The model under review builds one solid part; all positions refer to its coordinate system, in mm. A direction names the side the tool comes from. Coordinates: 2 decimals unless noted, no trailing zeros. Order: outer loops, then holes, each group sorted by start corner. A loop starts at its lowest first (then second) coordinate and runs counter-clockwise, first axis right, second up. Notation, with made-up numbers: (-9, -39.5) -> (5, -39.5) arc R13 ccw to (5, -27.5) -> close; hole circle Ø5 at (87, -24.5). An arc over 180 degrees is marked (long way). Answer as CSV lines item,"result". Start each with the question number.
from build123d import *
from OCP.BRepFilletAPI import BRepFilletAPI_MakeChamfer

# Parameters (mm, degrees)
SKETCH1_W           = 60
SKETCH1_H           = 45
BOSS_EXTRUDE1_DEPTH = 30
SKETCH2_W           = 8
SKETCH2_H           = 16
CUT_EXTRUDE1_DEPTH  = 20
CHAMFER1_SIZE       = 15
CHAMFER1_SIZE2      = 1.312329953
CHAMFER2_SIZE       = 5
CHAMFER2_SIZE2      = 5.958767963
CUT_EXTRUDE2_DEPTH  = 10


with BuildPart() as part:
    # Sketch1 → Boss-Extrude1 (new body)
    with BuildSketch(Plane(origin=(0, 0, 0), x_dir=(1, 0, 0), z_dir=(0, 1, 0))):
        with Locations((-30, 22.5)):
            Rectangle(SKETCH1_W, SKETCH1_H)
    extrude(amount=BOSS_EXTRUDE1_DEPTH)

    # Sketch2 → Cut-Extrude1 (cut)
    with BuildSketch(Plane(origin=(0, 0, 0), x_dir=(-1, 0, 0), z_dir=(0, -1, 0))):
        with Locations((47, 21)):
            Rectangle(SKETCH2_W, SKETCH2_H)
        with Locations((13, 21)):
            Rectangle(SKETCH2_W, SKETCH2_H)
    extrude(amount=-CUT_EXTRUDE1_DEPTH, mode=Mode.SUBTRACT)

    # Chamfer1: one chamfer whose edges measure the first distance from different faces: ONE call of the kernel's chamfer builder (chamfer() names one face for all edges)
    chamfer1_edges_1 = [part.edges().sort_by_distance(p)[0] for p in [
        (-51, 20, -21),
    ]]
    chamfer1_side_1 = [part.faces().sort_by_distance(p)[0] for p in [
        (-51, 10, -21),
    ]]
    chamfer1_edges_2 = [part.edges().sort_by_distance(p)[0] for p in [
        (-43, 20, -21),
    ]]
    chamfer1_side_2 = [part.faces().sort_by_distance(p)[0] for p in [
        (-43, 10, -21),
    ]]
    chamfer1_edges_3 = [part.edges().sort_by_distance(p)[0] for p in [
        (-17, 20, -21),
    ]]
    chamfer1_side_3 = [part.faces().sort_by_distance(p)[0] for p in [
        (-17, 10, -21),
    ]]
    chamfer1_edges_4 = [part.edges().sort_by_distance(p)[0] for p in [
        (-9, 20, -21),
    ]]
    chamfer1_side_4 = [part.faces().sort_by_distance(p)[0] for p in [
        (-9, 10, -21),
    ]]
    chamfer1 = BRepFilletAPI_MakeChamfer(part.part.solid().wrapped)
    for e in chamfer1_edges_1:
        chamfer1.Add(CHAMFER1_SIZE, CHAMFER1_SIZE2, e.wrapped, chamfer1_side_1[0].wrapped)  # the first distance lies on this face
    for e in chamfer1_edges_2:
        chamfer1.Add(CHAMFER1_SIZE, CHAMFER1_SIZE2, e.wrapped, chamfer1_side_2[0].wrapped)  # the first distance lies on this face
    for e in chamfer1_edges_3:
        chamfer1.Add(CHAMFER1_SIZE, CHAMFER1_SIZE2, e.wrapped, chamfer1_side_3[0].wrapped)  # the first distance lies on this face
    for e in chamfer1_edges_4:
        chamfer1.Add(CHAMFER1_SIZE, CHAMFER1_SIZE2, e.wrapped, chamfer1_side_4[0].wrapped)  # the first distance lies on this face
    add(Compound.cast(chamfer1.Shape()), mode=Mode.REPLACE)

    # Chamfer2: one chamfer whose edges measure the first distance from different faces: ONE call of the kernel's chamfer builder (chamfer() names one face for all edges)
    chamfer2_edges_1 = [part.edges().sort_by_distance(p)[0] for p in [
        (-13, 20, -29),
    ]]
    chamfer2_side_1 = [part.faces().sort_by_distance(p)[0] for p in [
        (-13, 9.298544625, -29),
    ]]
    chamfer2_edges_2 = [part.edges().sort_by_distance(p)[0] for p in [
        (-13, 20, -13),
    ]]
    chamfer2_side_2 = [part.faces().sort_by_distance(p)[0] for p in [
        (-13, 9.298544625, -13),
    ]]
    chamfer2_edges_3 = [part.edges().sort_by_distance(p)[0] for p in [
        (-47, 20, -29),
    ]]
    chamfer2_side_3 = [part.faces().sort_by_distance(p)[0] for p in [
        (-47, 9.298544625, -29),
    ]]
    chamfer2_edges_4 = [part.edges().sort_by_distance(p)[0] for p in [
        (-47, 20, -13),
    ]]
    chamfer2_side_4 = [part.faces().sort_by_distance(p)[0] for p in [
        (-47, 9.298544625, -13),
    ]]
    chamfer2 = BRepFilletAPI_MakeChamfer(part.part.solid().wrapped)
    for e in chamfer2_edges_1:
        chamfer2.Add(CHAMFER2_SIZE, CHAMFER2_SIZE2, e.wrapped, chamfer2_side_1[0].wrapped)  # the first distance lies on this face
    for e in chamfer2_edges_2:
        chamfer2.Add(CHAMFER2_SIZE, CHAMFER2_SIZE2, e.wrapped, chamfer2_side_2[0].wrapped)  # the first distance lies on this face
    for e in chamfer2_edges_3:
        chamfer2.Add(CHAMFER2_SIZE, CHAMFER2_SIZE2, e.wrapped, chamfer2_side_3[0].wrapped)  # the first distance lies on this face
    for e in chamfer2_edges_4:
        chamfer2.Add(CHAMFER2_SIZE, CHAMFER2_SIZE2, e.wrapped, chamfer2_side_4[0].wrapped)  # the first distance lies on this face
    add(Compound.cast(chamfer2.Shape()), mode=Mode.REPLACE)

    # Sketch4 → Cut-Extrude2 (cut)
    with BuildSketch(Plane(origin=(0, 0, -45), x_dir=(-1, 0, 0), z_dir=(0, 0, -1))):
        with BuildLine():
            Line((10, 0), (28.5, 0))
            ThreePointArc((28.5, 0), (34.073421984, 6.184666101), (42.397874378, 6.313583642))
            ThreePointArc((42.397874378, 6.313583642), (46.400635454, 7.606885175), (45.740315255, 11.761244612))
            ThreePointArc((45.740315255, 11.761244612), (24.568698428, 15.91316533), (10, 0))
        make_face()
    extrude(amount=-CUT_EXTRUDE2_DEPTH, mode=Mode.SUBTRACT)


solid = part.part
1) Consider section A-A (y = 8.25). Give the boundary of the cut face in (x, z).
2) Mouldability with a two-part tool opening along Y and no side actions: class faces 4 (the face through (-33.965, 6.134, -40.07)), 5 (the face through (-12.956, 17.535, -25.979)), 6 (the face through (-28, 9, -35)), 7 (the face through (-60, 15, -22)) as released by +Y, released by -Y, zero draft, split by the parting line, or undercut.
3) Wall thickness on L1, parallel to X at y = 7.5, z = -27; L2, parallel to Y at x = -11, z = -20; L3, parallel to Z at x = -49, y = 2.5: over which ranges is each line inside the solid? List them lowest first. Write a range as [from, to].
4) Tool access review of faces 1 (the face through (-30, 15, 0)), 2 (the face through (-46.367, 7.553, -40.07)), 3 (the face through (-51, 2, -21)): name each direction out of +Z, -Z, +X, -X, +Y, -Y from which nothing blocks a thin tool from reaching the whole face with its end or side.
5) Insertion check: pin 1 Ø3 at (x, y) = (-35, 9.5) entering from -Z. The pin has a flat end and moves straight along its axis. Give the tip position at first contact, or say it passes through.
6) Consider section D-D (z = -15.5). Give the boundary of the cut face in (x, y).
7) Consider section C-C (x = -35). Give the boundary of the cut face in (y, z), plus the area to 3 significant figures.
8) Consider section B-B (z = -20). Give the boundary of the cut face in (x, y), plus the area to 3 significant figures.
Result:
1,outline,"(-60, -45) -> (-46.7, -45) -> (-46.7, -35) -> (-13.86, -35) -> (-13.86, -45) -> (0, -45) -> (0, 0) -> (-60, 0) -> close; hole (-50.72, -29) -> (-43.28, -29) -> (-43.28, -13) -> (-50.72, -13) -> close; hole (-16.72, -29) -> (-9.28, -29) -> (-9.28, -13) -> (-16.72, -13) -> close"
2,face 4,"undercut"
2,face 5,"released by -Y"
2,face 6,"undercut"
2,face 7,"zero draft"
3,L1,"[-60, -50.78], [-43.22, -16.78], [-9.22, 0]"
3,L2,"[20, 30]"
3,L3,"[-45, -29], [-13, 0]"
4,face 1,"+Z, +X, -X, +Y, -Y"
4,face 2,"-Z"
4,face 3,"-Y"
5,pin 1,"z = -35"
6,outline,"(-60, 0) -> (-51, 0) -> (-51, 5) -> (-49.94, 17.1) -> (-44.06, 17.1) -> (-43, 5) -> (-43, 0) -> (-17, 0) -> (-17, 5) -> (-15.94, 17.1) -> (-10.06, 17.1) -> (-9, 5) -> (-9, 0) -> (0, 0) -> (0, 30) -> (-60, 30) -> close"
7,outline,"(0, -45) -> (6.55, -45) -> (6.55, -35) -> (16.73, -35) -> (16.73, -45) -> (30, -45) -> (30, 0) -> (0, 0) -> close"
7,area,"1,250 mm2"
8,outline,"(-60, 0) -> (-51, 0) -> (-51, 5) -> (-49.69, 20) -> (-44.31, 20) -> (-43, 5) -> (-43, 0) -> (-17, 0) -> (-17, 5) -> (-15.69, 20) -> (-10.31, 20) -> (-9, 5) -> (-9, 0) -> (0, 0) -> (0, 30) -> (-60, 30) -> close"
8,area,"1,520 mm2"
